from build123d import *

# Parameters (mm, degrees)
SKETCH1_R           = 5
BOSS_EXTRUDE1_DEPTH = 80
SKETCH2_R           = 6.5
BOSS_EXTRUDE2_DEPTH = 1
BOSS_EXTRUDE5_DEPTH = 5
SKETCH6_R           = 3.019653564
BOSS_EXTRUDE6_DEPTH = 7.5
BOSS_EXTRUDE7_DEPTH = 5
SKETCH8_R           = 3
BOSS_EXTRUDE8_DEPTH = 12.5
BOSS_EXTRUDE9_DEPTH = 5


with BuildPart() as part:
    # Sketch1 → Boss-Extrude1 (new body)
    with BuildSketch(Plane.XY):
        Circle(SKETCH1_R)
    extrude(amount=BOSS_EXTRUDE1_DEPTH)

    # Sketch2 → Boss-Extrude2 (add)
    with BuildSketch(Plane.XY.offset(80)):
        Circle(SKETCH2_R)
    extrude(amount=BOSS_EXTRUDE2_DEPTH)

    # Sketch5 → Boss-Extrude5 (add)
    with BuildSketch(Plane.XY.offset(81)):
        Polygon((4.778851136, -2.820156932), (4.831753114, 2.728528019), (0.052901978, 5.548684951), (-4.778851136, 2.820156932), (-4.831753114, -2.728528019), (-0.052901978, -5.548684951), align=None)
    extrude(amount=BOSS_EXTRUDE5_DEPTH)

    # Sketch6 → Boss-Extrude6 (add)
    with BuildSketch(Plane.XY.offset(86)):
        Circle(SKETCH6_R)
    extrude(amount=BOSS_EXTRUDE6_DEPTH)

    # Sketch7 → Boss-Extrude7 (add)
    with BuildSketch(Plane.XY.offset(93.5)):
        Polygon((4.778851136, -2.820156932), (4.831753114, 2.728528019), (0.052901978, 5.548684951), (-4.778851136, 2.820156932), (-4.831753114, -2.728528019), (-0.052901978, -5.548684951), align=None)
    extrude(amount=BOSS_EXTRUDE7_DEPTH)

    # Sketch8 → Boss-Extrude8 (add)
    with BuildSketch(Plane.XY.offset(98.5)):
        Circle(SKETCH8_R)
    extrude(amount=BOSS_EXTRUDE8_DEPTH)

    # Sketch9 → Boss-Extrude9 (add)
    with BuildSketch(Plane.XY.offset(111)):
        Polygon((4.778851136, -2.820156932), (4.831753114, 2.728528019), (0.052901978, 5.548684951), (-4.778851136, 2.820156932), (-4.831753114, -2.728528019), (-0.052901978, -5.548684951), align=None)
    extrude(amount=BOSS_EXTRUDE9_DEPTH)


solid = part.part
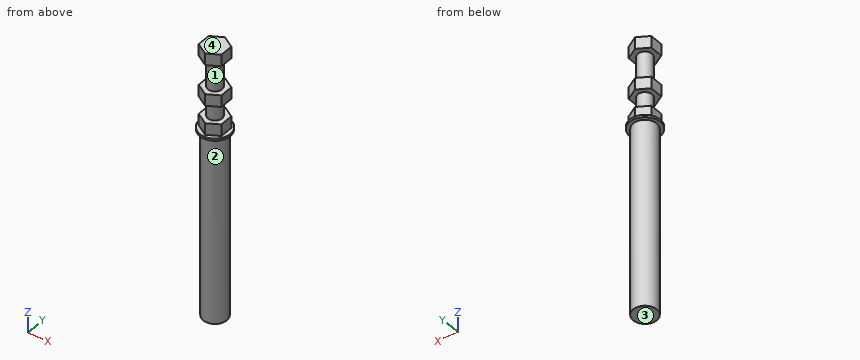
Read the model definition and answer for the solid it produces. Units are mm, in the model's axes. Face numbers are marked on the shaded views. Round coordinates to 2 decimals unless told otherwise and drop trailing zeros. Write each loop counter-clockwise with the first axis right and the second up, starting at its lowest first coordinate (ties: lowest second). Pieces come first, ordered by that corner, then holes.
1. The part is cut by section C-C, the plane x = -1.75. Determine the outline of the cut face in (y, z), then the cut area to 3 significant figures.
2. The part is cut by section B-B, the plane y = -1.25. Determine the outline of the cut face in (x, z).
3. Given pin 1 Ø1 at (x, y) = (3.5, 5) entering from +Z; pin 2 Ø1.5 at (y, z) = (1, 52) entering from -X; pin 3 Ø4 at (x, z) = (3.5, 44.5) entering from +Y; pin 4 Ø6.5 at (x, y) = (0.5, 2) entering from -Z, each flat-ended and moving along its own axis, determine where each tip first touches the part or whether it passes through.
4. The part is cut by section D-D, the plane z = 48.5. Determine the outline of the cut face in (x, y), then the cut area to 3 significant figures.
5. Straight lines are drawn through the part: L1, parallel to Z at x = -3, y = 1.75; L2, parallel to Z at x = 5.5, y = -3.25; L3, parallel to Y at x = 0, z = 72. For each, find the intervals that lie inside material, in ascending order.
6. The part is cut by section A-A, the plane z = 100. Determine the outline of the cut face in (x, y).
7. Determine the mould class of the marked faces 1, 2, 3 and 4 for opening direction Z: pulls with the +Z half, pulls with the -Z half, needs draft (parallel to the pull), parting line crosses it, or undercut.
Values:
1. outline: (-6.26, 80) - (-4.68, 80) - (-4.68, 0) - (4.68, 0) - (4.68, 80) - (6.26, 80) - (6.26, 81) - (4.53, 81) - (4.53, 86) - (2.46, 86) - (2.46, 93.5) - (4.53, 93.5) - (4.53, 98.5) - (2.44, 98.5) - (2.44, 111) - (4.53, 111) - (4.53, 116) - (-4.55, 116) - (-4.55, 111) - (-2.44, 111) - (-2.44, 98.5) - (-4.55, 98.5) - (-4.55, 93.5) - (-2.46, 93.5) - (-2.46, 86) - (-4.55, 86) - (-4.55, 81) - (-6.26, 81) - close
1. area: 996 mm2
2. outline: (-6.38, 80) - (-4.84, 80) - (-4.84, 0) - (4.84, 0) - (4.84, 80) - (6.38, 80) - (6.38, 81) - (4.79, 81) - (4.79, 86) - (2.75, 86) - (2.75, 93.5) - (4.79, 93.5) - (4.79, 98.5) - (2.73, 98.5) - (2.73, 111) - (4.79, 111) - (4.79, 116) - (-4.82, 116) - (-4.82, 111) - (-2.73, 111) - (-2.73, 98.5) - (-4.82, 98.5) - (-4.82, 93.5) - (-2.75, 93.5) - (-2.75, 86) - (-4.82, 86) - (-4.82, 81) - (-6.38, 81) - close
3. pin 1: stops at z = 81
3. pin 2: stops at x = -4.99
3. pin 3: stops at y = 4.77
3. pin 4: stops at z = 0
4. outline: circle Ø10 at (0, 0)
4. area: 78.5 mm2
5. L1: z = 0 to 86, 93.5 to 98.5, 111 to 116
5. L2: z = 80 to 81
5. L3: y = -5 to 5
6. outline: circle Ø6 at (0, 0)
7. face 1: undercut
7. face 2: needs draft
7. face 3: pulls with the -Z half
7. face 4: pulls with the +Z half
